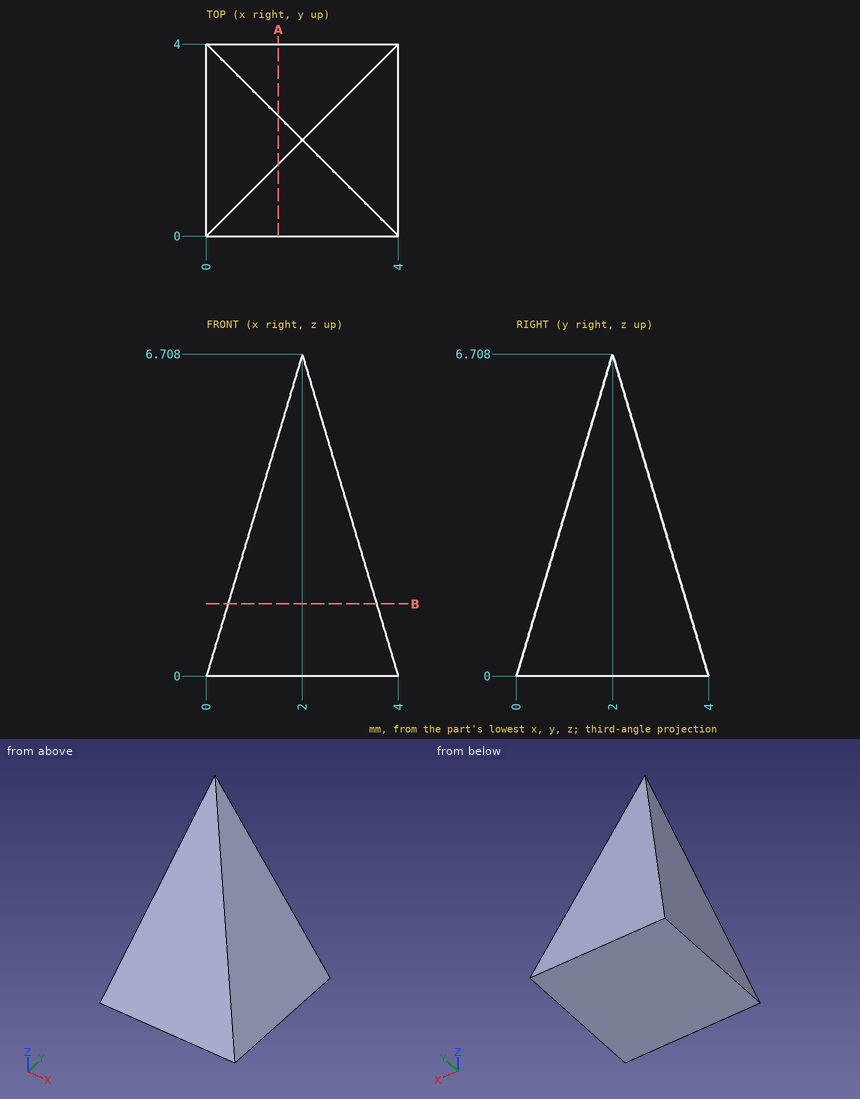
Input: dimensioned drawing with shaded views. Units: mm. Origin: part minimum x, y, z. Coordinates: 2 decimals unless noted, no trailing zeros. Loops run counter-clockwise (first coordinate to the right, second up) from the corner with the lowest first, then second, coordinate; pieces in that order, holes last. Notation, with made-up numbers: (40, 24.25) -> (98, 24.25) arc R22 ccw to (98, 41.25) -> close; hole circle Ø2 at (48.5, 64). An arc over 180 degrees is marked (long way). Use a Markdown table: item, result. Add a question column.
(1) Line query: line 1 along X through (y, z) = (3.05, 2); line 2 along Y through (x, z) = (2.25, 1.25); line 3 along X through (y, z) = (2.15, 5.5). Output: solid intervals per line, ascending.
(2) Pin query (flat end, axial travel): pin 1 Ø1 at (y, z) = (2.5, 5.5) entering from +X. Return the tip coordinate at first contact, or that it passes through.
(3) Section query B-B, the plane z = 1.5. Return loops of the section in (x, y).
(4) Section query A-A, the plane x = 1.5. Return loops of the section in (y, z).
Answer:
| question | item | result |
|---|---|---|
| 1 | line 1 | x = 0.6 to 3.4 |
| 1 | line 2 | y = 0.37 to 3.63 |
| 1 | line 3 | x = 1.64 to 2.36 |
| 2 | pin 1 | stops at x = 2.51 |
| 3 | outline | (0.45, 0.45) -> (3.55, 0.45) -> (3.55, 3.55) -> (0.45, 3.55) -> close |
| 4 | outline | (0, 0) -> (4, 0) -> (2.5, 5.03) -> (1.5, 5.03) -> close |
